Verification items for the finished model (mm, model axes). A direction names the side the tool comes from. Give positions to 0.01 mm unless a question says otherwise; leave off trailing zeros. Loops run counter-clockwise (first coordinate to the right, second up) from the corner with the lowest first, then second, coordinate; pieces in that order, holes last. Notation, with made-up numbers: (42.25, -14.5) -> (89.25, -14.5) arc R20 cw to (89.25, -7.5) -> close; hole circle Ø11 at (-3.5, 84). An arc over 180 degrees is marked (long way). Use one line per item in the form item = value. Start each with the question number.
Autodesk Inventor part; units mm, degrees
ref_plane "YZ Plane" through (0, 0, 0) normal (1, 0, 0) x (0, 1, 0)
ref_plane "XZ Plane" through (0, 0, 0) normal (0, 1, 0) x (-1, 0, 0)
ref_plane "XY Plane" through (0, 0, 0) normal (0, 0, 1) x (1, 0, 0)
sketch "Sketch1" plane through (0, 0, 0) normal (0, 1, 0) x (-1, 0, 0)
  line L0 (-60, -15) -> (60, -15)
  line L1 (60, -15) -> (60, 15)
  line L2 (60, 15) -> (-60, 15)
  line L3 (-60, 15) -> (-60, -15)
  line L4 (-60, -15) -> (60, 15) construction
  line L5 (60, -15) -> (-60, 15) construction
  circle A0 centre (-60, 0) radius 15
  circle A1 centre (60, 0) radius 15
  point P0 (0, 0)
  dimension "d0" = 120
  dimension "d1" = 30
extrude "Extrusion1" add sketch "Sketch1" along normal mid plane 12
sketch "Sketch2" plane through (0, 6, 0) normal (0, 1, 0) x (1, 0, 0)
  point P0 (0, 0)
sketch "Sketch3" plane through (0, 0, 0) normal (0, 1, 0) x (-1, 0, 0)
  circle A0 centre (60, 0) radius 15
  circle A1 centre (60, 0) radius 10
  point P0 (0, 0)
  dimension "d4" = 20
extrude "Extrusion2" add sketch "Sketch3" along normal mid plane 32
sketch "Sketch4" plane through (0, 0, 0) normal (0, 1, 0) x (-1, 0, 0)
  circle A0 centre (-60, 0) radius 15
  circle A1 centre (-60, 0) radius 10
  point P0 (0, 0)
  dimension "d7" = 20
extrude "Extrusion3" add sketch "Sketch4" along normal mid plane 14
sketch "Sketch5" plane through (0, 0, 0) normal (0, 1, 0) x (-1, 0, 0)
  point P0 (0, 0)
hole "Hole1" at (-60, 6, 0) direction (0, -1, 0) diameter 20 end through all
hole "Hole2" at (60, 6, 0) direction (0, -1, 0) diameter 20 end through all
sketch "Sketch6" plane through (0, 6, 0) normal (0, 1, 0) x (1, 0, 0)
  arc A0 (-48.8197, -10) -> (-48.8197, 10) centre (-60, 0) ccw
  arc A1 (48.8197, 10) -> (48.8197, -10) centre (60, 0) ccw
  circle A2 centre (-60, 0) radius 10
  line L0 (48.8197, 10) -> (-48.8197, 10)
  line L1 (-60, 10) -> (-60, -10)
  line L2 (-48.8197, -10) -> (48.8197, -10)
  line L3 (60, -10) -> (60, 10)
  line L4 (60, 10) -> (-60, -10) construction
  line L5 (-60, 10) -> (60, -10) construction
  point P0 (0, 0)
  dimension "d28" = 30
extrude "Extrusion4" cut sketch "Sketch6" against normal blind 2 contours A0 L0 A1 L2
mirror "Mirror1" about plane through (0, 0, 0) normal (0, 1, 0) of "Extrusion4"
properties part number "connecting_link"
Item 1: Material ranges on line 1 (Z direction, x = -27.5, y = -5.5); line 2 (X direction, y = -5, z = 3.75); line 3 (Y direction, x = -9.5, z = -10.75), recorded low to high.
Item 2: Sectioned sample at B-B, the plane x = 19. Enter the section's corners in (y, z).
Item 3: Sectioned sample at C-C, the plane y = -13. Enter the section's corners in (x, z).
Item 4: Gauge pin test, flat ends, axial feed: pin 1 Ø4 at (x, z) = (15.5, -12.5) entering from +Y; pin 2 Ø5.5 at (x, z) = (-10.5, 13) entering from -Y; pin 3 Ø12 at (x, z) = (-60, 0) entering from +Y; pin 4 Ø5 at (y, z) = (0, 8) entering from +X. Record the tip position at first contact, or that the pin passes through.
Item 5: Draft check along Z on faces 1 (the flat face through (-1, 0, 15)), 2 (the cylindrical face through (45, 5, 0)), 3 (the flat face through (-70, -16, -3)). Enter one of: +Z half, -Z half, draft (parallel to the pull), parting line (faces both ways), or undercut.
Item 6: Tool access check on faces 4 (the cylindrical face through (-63.722, -0.224, 9.282)), 5 (the cylindrical face through (-74.307, 0.224, 4.506)), 6 (the flat face through (50, 7, -3)). Record the directions out of +Z, -Z, +X, -X, +Y, -Y that give a thin tool (end or side, any length) a straight path to the whole face; none if there is none.
Outcome:
q1.line_1 = -15 to -10, 10 to 15
q1.line_2 = -74.52 to -69.27, -50.73 to -45.48, 45.48 to 50.73, 69.27 to 74.52
q1.line_3 = -6 to 6
q2.outline = (-6, -15) -> (6, -15) -> (6, -10) -> (4, -10) -> (4, 10) -> (6, 10) -> (6, 15) -> (-6, 15) -> (-6, 10) -> (-4, 10) -> (-4, -10) -> (-6, -10) -> close
q3.outline = circle Ø30 at (-60, 0); hole circle Ø20 at (-60, 0)
q4.pin_1 = 6
q4.pin_2 = -6
q4.pin_3 = through
q4.pin_4 = 73.96
q5.face_1 = +Z half
q5.face_2 = undercut
q5.face_3 = draft
q6.face_4 = +Y, -Y
q6.face_5 = none
q6.face_6 = +Z, -Z, +X, +Y
